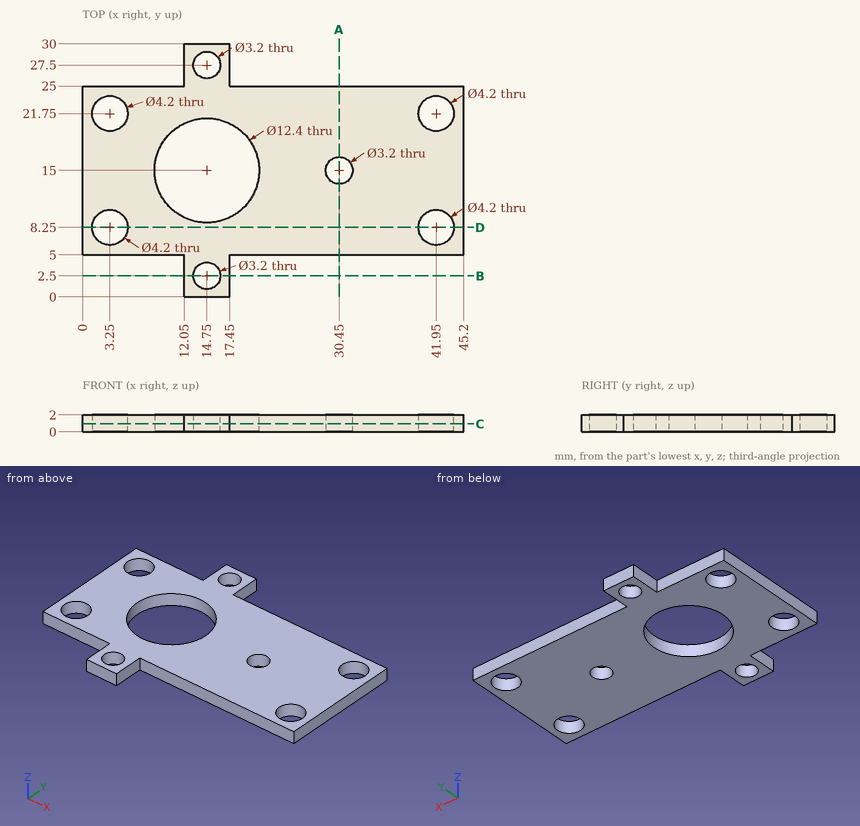
Answer from the drawing. Dimensions are ordinates in mm from the lowest x, y and z of the part. Coordinates: 2 decimals unless noted, no trailing zeros. Order: outer loops, then holes, each group sorted by start corner. A loop starts at its lowest first (then second) coordinate and runs counter-clockwise, first axis right, second up. Notation, with made-up numbers: (-8.75, -11) - (36.25, -11) arc R24 ccw to (36.25, -1) - close; hole circle Ø9 at (35.25, 34.5). An arc over 180 degrees is marked (long way). Use one line per item in the form item = value.
(1) Section C-C, the plane z = 0.95 is taken. Give the number of separate pieces and of enclosed holes in the cut face, then the cut area to 3 significant figures.
Computed values:
separate_pieces = 1
enclosed_holes = 8
area = 758 mm²
(2) Section D-D, the plane y = 8.25 is taken. Give the vertices of the cut face in (x, z), then the cut area to 3 significant figures.
Computed values:
outline = (0, 0) - (1.15, 0) - (1.15, 2) - (0, 2) - close; (5.35, 0) - (39.85, 0) - (39.85, 2) - (5.35, 2) - close; (44.05, 0) - (45.2, 0) - (45.2, 2) - (44.05, 2) - close
area = 73.6 mm²
(3) Straight lines are drawn through the part: L1, parallel to X at y = 21.75, z = 0.8; L2, parallel to Y at x = 14.75, z = 1; L3, parallel to Y at x = 13.5, z = 0.5. For each, find the intervals that lie inside material, in ascending order.
Computed values:
L1 = 0 to 1.15, 5.35 to 39.85, 44.05 to 45.2
L2 = 0 to 0.9, 4.1 to 8.8, 21.2 to 25.9, 29.1 to 30
L3 = 0 to 1.5, 3.5 to 8.93, 21.07 to 26.5, 28.5 to 30
(4) Given pin 1 Ø5 at (x, y) = (3.25, 21.75) entering from +Z; pin 2 Ø1 at (x, z) = (6.5, 0.5) entering from +Y; pin 3 Ø1 at (y, z) = (28.5, 1) entering from -X, each flat-ended and moving along its own axis, determine where each tip first touches the part or whether it passes through.
Computed values:
pin_1 = 2
pin_2 = 25
pin_3 = 12.05
(5) Section A-A, the plane x = 30.45 is taken. Give the vertices of the cut face in (y, z), then the cut area to 3 significant figures.
Computed values:
outline = (5, 0) - (13.4, 0) - (13.4, 2) - (5, 2) - close; (16.6, 0) - (25, 0) - (25, 2) - (16.6, 2) - close
area = 33.6 mm²
(6) Section B-B, the plane y = 2.5 is taken. Give the vertices of the cut face in (x, z), then the cut area to 3 significant figures.
Computed values:
outline = (12.05, 0) - (13.15, 0) - (13.15, 2) - (12.05, 2) - close; (16.35, 0) - (17.45, 0) - (17.45, 2) - (16.35, 2) - close
area = 4.40 mm²
